```python
from build123d import *

# Parameters (mm, degrees)
SKETCH1_W                            = 38.1
SKETCH1_H                            = 30.48
BOSS_EXTRUDE1_DEPTH                  = 2.54
F_48_0_076_DIAMETER_HOLE1_AT_2_COUNT = 2
F_48_0_076_DIAMETER_HOLE1_AT_2_PITCH = 2.54
F_48_0_076_DIAMETER_HOLE1_AT_3_COUNT = 2
F_48_0_076_DIAMETER_HOLE1_AT_3_PITCH = 2.54
CIRPATTERN1_COUNT                    = 4
F_4_CLEARANCE_HOLE3_AT_2_COUNT       = 2
F_4_CLEARANCE_HOLE3_AT_2_PITCH       = 30.48
F_4_CLEARANCE_HOLE3_AT_3_COUNT       = 2
F_4_CLEARANCE_HOLE3_AT_3_PITCH       = 38.1
F_4_CLEARANCE_HOLE3_AT_4_COUNT       = 2
F_4_CLEARANCE_HOLE3_AT_4_PITCH       = 22.86
SKETCH10_W                           = 7.4676
SKETCH10_H                           = 7.5438
CUT_EXTRUDE1_DEPTH                   = 3.54
FILLET1_R                            = 0.79375
CUT_EXTRUDE2_DEPTH                   = 3.54


with BuildPart() as part:
    # Sketch1 → Boss-Extrude1 (new body)
    with BuildSketch(Plane.XY):
        Rectangle(SKETCH1_W, SKETCH1_H)
    extrude(amount=-BOSS_EXTRUDE1_DEPTH)

    # Sketch2 → 48 _0.076_ Diameter Hole1 (revolve, cut)
    with BuildSketch(Plane(origin=(0, 5.08, 0), x_dir=(0, -1, 0), z_dir=(1, 0, 0))):
        Polygon((0, 0), (0, 2.54), (1.0795, 2.54), (0.9652, 2.4257), (0.9652, 0.1143), (1.0795, 0), align=None)
    f_48_0_076_diameter_hole1 = revolve(axis=Axis((0, 5.08, 6.35), (0, 0, -1)), mode=Mode.SUBTRACT)

    # 48 _0.076_ Diameter Hole1 at 2: 48 _0.076_ Diameter Hole1 ×2
    with Locations(*[(i * F_48_0_076_DIAMETER_HOLE1_AT_2_PITCH, 0, 0) for i in range(1, F_48_0_076_DIAMETER_HOLE1_AT_2_COUNT)]):
        add(f_48_0_076_diameter_hole1, mode=Mode.SUBTRACT)

    # 48 _0.076_ Diameter Hole1 at 3: 48 _0.076_ Diameter Hole1 ×2
    with Locations(*[(-i * F_48_0_076_DIAMETER_HOLE1_AT_3_PITCH, 0, 0) for i in range(1, F_48_0_076_DIAMETER_HOLE1_AT_3_COUNT)]):
        add(f_48_0_076_diameter_hole1, mode=Mode.SUBTRACT)

    # Sketch4 → 4 Clearance Hole4 (revolve, cut)
    with BuildSketch(Plane(origin=(0, 10.668, 0), x_dir=(0, -1, 0), z_dir=(1, 0, 0))):
        Polygon((0, 0), (0, 2.54), (1.778, 2.54), (1.63195, 2.39395), (1.63195, 0.14605), (1.778, 0), align=None)
    f_4_clearance_hole4 = revolve(axis=Axis((0, 10.668, 6.35), (0, 0, -1)), mode=Mode.SUBTRACT)

    # CirPattern1: 48 _0.076_ Diameter Hole1, 4 Clearance Hole4 ×4 about axis
    cirpattern1_axis = Axis((0, 0, 0), (0, 0, 1))
    add([f_48_0_076_diameter_hole1.rotate(cirpattern1_axis, i * 360 / CIRPATTERN1_COUNT) for i in range(1, CIRPATTERN1_COUNT)], mode=Mode.SUBTRACT)
    add([f_4_clearance_hole4.rotate(cirpattern1_axis, i * 360 / CIRPATTERN1_COUNT) for i in range(1, CIRPATTERN1_COUNT)], mode=Mode.SUBTRACT)

    # CirPattern1 copy 1 sketch → CirPattern1 copy 1 (revolve, cut)
    with BuildSketch(Plane(origin=(-5.08, 2.54, 0), x_dir=(1, 0, 0), z_dir=(0, 1, 0))):
        Polygon((0, 0), (0, 2.54), (1.0795, 2.54), (0.9652, 2.4257), (0.9652, 0.1143), (1.0795, 0), align=None)
    revolve(axis=Axis((-5.08, 2.54, 6.35), (0, 0, -1)), mode=Mode.SUBTRACT)

    # CirPattern1 copy 2 sketch → CirPattern1 copy 2 (revolve, cut)
    with BuildSketch(Plane(origin=(-2.54, -5.08, 0), x_dir=(0, 1, 0), z_dir=(-1, 0, 0))):
        Polygon((0, 0), (0, 2.54), (1.0795, 2.54), (0.9652, 2.4257), (0.9652, 0.1143), (1.0795, 0), align=None)
    revolve(axis=Axis((-2.54, -5.08, 6.35), (0, 0, -1)), mode=Mode.SUBTRACT)

    # CirPattern1 copy 3 sketch → CirPattern1 copy 3 (revolve, cut)
    with BuildSketch(Plane(origin=(5.08, -2.54, 0), x_dir=(-1, 0, 0), z_dir=(0, -1, 0))):
        Polygon((0, 0), (0, 2.54), (1.0795, 2.54), (0.9652, 2.4257), (0.9652, 0.1143), (1.0795, 0), align=None)
    revolve(axis=Axis((5.08, -2.54, 6.35), (0, 0, -1)), mode=Mode.SUBTRACT)

    # CirPattern1 copy 4 sketch → CirPattern1 copy 4 (revolve, cut)
    with BuildSketch(Plane(origin=(-5.08, -2.54, 0), x_dir=(1, 0, 0), z_dir=(0, 1, 0))):
        Polygon((0, 0), (0, 2.54), (1.0795, 2.54), (0.9652, 2.4257), (0.9652, 0.1143), (1.0795, 0), align=None)
    revolve(axis=Axis((-5.08, -2.54, 6.35), (0, 0, -1)), mode=Mode.SUBTRACT)

    # CirPattern1 copy 5 sketch → CirPattern1 copy 5 (revolve, cut)
    with BuildSketch(Plane(origin=(2.54, -5.08, 0), x_dir=(0, 1, 0), z_dir=(-1, 0, 0))):
        Polygon((0, 0), (0, 2.54), (1.0795, 2.54), (0.9652, 2.4257), (0.9652, 0.1143), (1.0795, 0), align=None)
    revolve(axis=Axis((2.54, -5.08, 6.35), (0, 0, -1)), mode=Mode.SUBTRACT)

    # CirPattern1 copy 6 sketch → CirPattern1 copy 6 (revolve, cut)
    with BuildSketch(Plane(origin=(5.08, 2.54, 0), x_dir=(-1, 0, 0), z_dir=(0, -1, 0))):
        Polygon((0, 0), (0, 2.54), (1.0795, 2.54), (0.9652, 2.4257), (0.9652, 0.1143), (1.0795, 0), align=None)
    revolve(axis=Axis((5.08, 2.54, 6.35), (0, 0, -1)), mode=Mode.SUBTRACT)

    # Sketch8 → 4 Clearance Hole3 (revolve, cut)
    with BuildSketch(Plane(origin=(-15.24, 11.43, 0), x_dir=(0, -1, 0), z_dir=(1, 0, 0))):
        Polygon((0, 0), (0, 2.54), (1.778, 2.54), (1.63195, 2.39395), (1.63195, 0.14605), (1.778, 0), align=None)
    f_4_clearance_hole3 = revolve(axis=Axis((-15.24, 11.43, 6.35), (0, 0, -1)), mode=Mode.SUBTRACT)

    # 4 Clearance Hole3 at 2: 4 Clearance Hole3 ×2
    with Locations(*[(i * F_4_CLEARANCE_HOLE3_AT_2_PITCH, 0, 0) for i in range(1, F_4_CLEARANCE_HOLE3_AT_2_COUNT)]):
        add(f_4_clearance_hole3, mode=Mode.SUBTRACT)

    # 4 Clearance Hole3 at 3: 4 Clearance Hole3 ×2
    with Locations(*[Vector(0.8, -0.6, 0) * (i * F_4_CLEARANCE_HOLE3_AT_3_PITCH) for i in range(1, F_4_CLEARANCE_HOLE3_AT_3_COUNT)]):
        add(f_4_clearance_hole3, mode=Mode.SUBTRACT)

    # 4 Clearance Hole3 at 4: 4 Clearance Hole3 ×2
    with Locations(*[(0, -i * F_4_CLEARANCE_HOLE3_AT_4_PITCH, 0) for i in range(1, F_4_CLEARANCE_HOLE3_AT_4_COUNT)]):
        add(f_4_clearance_hole3, mode=Mode.SUBTRACT)

    # Sketch10 → Cut-Extrude1 (cut, through all)
    with BuildSketch(Plane(origin=(0, 0, -2.54), x_dir=(-1, 0, 0), z_dir=(0, 0, -1))):
        with Locations((8.9662, 9.5123)):
            Rectangle(SKETCH10_W, SKETCH10_H)
    extrude(amount=-CUT_EXTRUDE1_DEPTH, mode=Mode.SUBTRACT)

    # Fillet1
    fillet1_edges = [part.edges().sort_by_distance(p)[0] for p in [
        (-12.7, 13.2842, -1.27),
        (-12.7, 5.7404, -1.27),
        (-5.2324, 5.7404, -1.27),
        (-5.2324, 13.2842, -1.27),
        (19.05, -15.24, -1.27),
        (-19.05, -15.24, -1.27),
        (-19.05, 15.24, -1.27),
        (19.05, 15.24, -1.27),
    ]]
    fillet(fillet1_edges, radius=FILLET1_R)

    # Sketch11 → Cut-Extrude2 (cut, through all)
    with BuildSketch(Plane.XY):
        with BuildLine():
            Line((5.619985846, -4.721960234), (7.256475174, -6.358449562))
            ThreePointArc((7.256475174, -6.358449562), (7.256475174, -7.256475174), (6.358449562, -7.256475174))
            Line((6.358449562, -7.256475174), (4.721960234, -5.619985846))
            ThreePointArc((4.721960234, -5.619985846), (4.721960234, -4.721960234), (5.619985846, -4.721960234))
        make_face()
    extrude(amount=-CUT_EXTRUDE2_DEPTH, mode=Mode.SUBTRACT)


solid = part.part
```
The model under review builds one solid part; all positions refer to its coordinate system, in mm. Coordinates: 2 decimals unless noted, no trailing zeros. Write each loop counter-clockwise with the first axis right and the second up, starting at its lowest first coordinate (ties: lowest second). Pieces come first, ordered by that corner, then holes.
1) We need section B-B on y = -2.54. State the section outline as (x, z) points, then the cut area to 3 significant figures.
2) To check wall thickness, follow probe 1 along X at (y, z) = (5.08, -0.75); probe 2 along Y at (x, z) = (5.08, -1.05); probe 3 along Y at (x, z) = (-9.5, -1.5). State the ranges of each line that lie inside material, in increasing order.
3) We need section D-D on z = -1. Count the separate pieces of the cut face and the enclosed holes in it, then the cut area to 3 significant figures.
4) Clearance check with flat-ended pins moving along their axes: pin 1 Ø2 at (x, y) = (2.54, 5.08) entering from +Z; pin 2 Ø1.2 at (x, y) = (-2.54, 5.08) entering from -Z (3 decimals). State where each tip first meets the part, or that it passes through.
5) We need section C-C on y = 5.08. State the section outline as (x, z) points, then the cut area to 3 significant figures.
6) We need section A-A on x = -2.54. State the section outline as (y, z) points.
7) The part is to be moulded in two halves that separate along Y. For faces 1 (the face through (-6.044, -0.042, -1.254)), 2 (the face through (0, 0, 0)), 3 (the face through (-12.7, 9, -1)), say which applies: pulls with the +Y half, pulls with the -Y half, needs draft (parallel to the pull), parting line crosses it, or undercut.
Answer list:
1. outline: (-19.05, -2.54) - (-6.16, -2.54) - (-6.05, -2.43) - (-6.05, -0.11) - (-6.16, 0) - (-19.05, 0) - close; (-4.11, -2.43) - (-4, -2.54) - (4, -2.54) - (4.11, -2.43) - (4.11, -0.11) - (4, 0) - (-4, 0) - (-4.11, -0.11) - close; (6.05, -2.43) - (6.16, -2.54) - (19.05, -2.54) - (19.05, 0) - (6.16, 0) - (6.05, -0.11) - close
1. area: 86.9 mm2
2. probe 1: x = -19.05 to -3.51, -1.57 to -0.97, 0.97 to 1.57, 3.51 to 19.05
2. probe 2: y = -15.24 to -5.98, -4.54 to -3.51, -1.57 to -0.97, 0.97 to 1.57, 3.51 to 15.24
2. probe 3: y = -15.24 to -1.14, 1.14 to 5.74, 13.28 to 15.24
3. separate pieces: 1
3. enclosed holes: 22
3. area: 999 mm2
4. pin 1: stops at z = -0.08
4. pin 2: passes through
5. outline: (-19.05, -2.54) - (-3.62, -2.54) - (-3.51, -2.43) - (-3.51, -0.11) - (-3.62, 0) - (-19.05, 0) - close; (-1.57, -2.43) - (-1.46, -2.54) - (-1.08, -2.54) - (-0.97, -2.43) - (-0.97, -0.11) - (-1.08, 0) - (-1.46, 0) - (-1.57, -0.11) - close; (0.97, -2.43) - (1.08, -2.54) - (1.46, -2.54) - (1.57, -2.43) - (1.57, -0.11) - (1.46, 0) - (1.08, 0) - (0.97, -0.11) - close; (3.51, -2.43) - (3.62, -2.54) - (19.05, -2.54) - (19.05, 0) - (3.62, 0) - (3.51, -0.11) - close
5. area: 82.0 mm2
6. outline: (-15.24, -2.54) - (-6.16, -2.54) - (-6.05, -2.43) - (-6.05, -0.11) - (-6.16, 0) - (-15.24, 0) - close; (-4.11, -2.43) - (-4, -2.54) - (4, -2.54) - (4.11, -2.43) - (4.11, -0.11) - (4, 0) - (-4, 0) - (-4.11, -0.11) - close; (6.05, -2.43) - (6.16, -2.54) - (15.24, -2.54) - (15.24, 0) - (6.16, 0) - (6.05, -0.11) - close
7. face 1: undercut
7. face 2: needs draft
7. face 3: undercut
